```python
from build123d import *

# Parameters (mm, degrees)
F0_W     = 152.4
F0_H     = 177.8
F1_DEPTH = 88.9
F2_SIZE2 = 69.85
F2_SIZE  = 101.6
F3_W     = 127
F3_H     = 63.5
F4_DEPTH = 76.2


with BuildPart() as f1:
    # F0 (on Top) → F1 (new body)
    with BuildSketch(Plane.XY):
        with Locations((1.3535544276, 18.5724278663)):
            Rectangle(F0_W, F0_H)
    extrude(amount=F1_DEPTH)

    # F2
    f2_edges = [f1.edges().sort_by_distance(p)[0] for p in [
        (1.353554, -70.327572, 88.9),
    ]]
    f2_side = f1.faces().sort_by_distance((1.353554, 18.572428, 88.9))[0]
    chamfer(f2_edges, length=F2_SIZE, length2=F2_SIZE2, reference=f2_side)

    # F3 (on face) → F4 (cut)
    with BuildSketch(Plane(origin=(0, 107.4724278663, 0), x_dir=(-1, 0, 0), z_dir=(0, 1, 0))):
        with Locations((-1.3535544276, 44.45)):
            Rectangle(F3_W, F3_H)
    extrude(amount=-F4_DEPTH, mode=Mode.SUBTRACT)


solid = f1.part
```
Model file for the job. Use its own axes, mm. A direction names the side the tool comes from. Give positions to 0.01 mm unless a question says otherwise; leave off trailing zeros. Loops run counter-clockwise (first coordinate to the right, second up) from the corner with the lowest first, then second, coordinate; pieces in that order, holes last. Notation, with made-up numbers: (35.5, 49) -> (51.5, 49) arc R6 ccw to (51.5, 55) -> close; hole circle Ø9 at (73, -8). An arc over 180 degrees is marked (long way). Use CSV: the item, a comma, the result in double quotes. Start each with the question number.
1) Tool access for faces 1 (the flat face through (0, 20, 0)), 2 (the flat face through (2, 70, 76.2)): list every direction of +Z, -Z, +X, -X, +Y, -Y with a clear straight run to the whole face (end or side of a thin tool).
2) Slice it at C-C on z = 21.5. Give the cut face in (x, y).
3) Flat gauge pins, fed straight in: pin 1 Ø6 at (x, z) = (45.5, 78) entering from -Y; pin 2 Ø12 at (x, y) = (-6, -52.5) entering from +Z; pin 3 Ø10 at (x, y) = (20, -21) entering from -Z. Where does each tip first touch, or does it go through?
4) Slice it at A-A on y = 87.5. Give the cut face in (x, z), plus the area to 3 significant figures.
5) Wall check: line 1 (Z direction, x = -36, y = 99); line 2 (X direction, y = 76.5, z = 30.5); line 3 (Y direction, x = 31, z = 23). Give the ranges that are in metal, low to high.
6) Slice it at B-B on x = -29. Give the cut face in (y, z), plus the area to 3 significant figures.
7) Mould opens along X. For faces 3 (the flat face through (2, 31.272, 45)), 4 (the flat face through (0, 107.472, 4)), 5 (the flat face through (77.554, 37, 34)) say: released by +X, released by -X, zero draft, split by the parting line, or undercut.
8) Slice it at D-D on y = 27. Give the cut face in (x, z).
Computed values:
1,face 1,"-Z, +X, -X, +Y, -Y"
1,face 2,"+Y"
2,outline,"(-74.85, -66.76) -> (77.55, -66.76) -> (77.55, 107.47) -> (64.85, 107.47) -> (64.85, 31.27) -> (-62.15, 31.27) -> (-62.15, 107.47) -> (-74.85, 107.47) -> close"
3,pin 1,"stops at y = 11.05"
3,pin 2,"stops at z = 35.43"
3,pin 3,"stops at z = 0"
4,outline,"(-74.85, 0) -> (77.55, 0) -> (77.55, 88.9) -> (-74.85, 88.9) -> close; hole (-62.15, 12.7) -> (64.85, 12.7) -> (64.85, 76.2) -> (-62.15, 76.2) -> close"
4,area,"5,480 mm^2"
5,line 1,"z = 0 to 12.7, 76.2 to 88.9"
5,line 2,"x = -74.85 to -62.15, 64.85 to 77.55"
5,line 3,"y = -64.58 to 31.27"
6,outline,"(-70.33, 0) -> (107.47, 0) -> (107.47, 12.7) -> (31.27, 12.7) -> (31.27, 76.2) -> (107.47, 76.2) -> (107.47, 88.9) -> (31.27, 88.9) -> (-70.33, 19.05) -> close"
6,area,"7,420 mm^2"
7,face 3,"undercut"
7,face 4,"zero draft"
7,face 5,"released by +X"
8,outline,"(-74.85, 0) -> (77.55, 0) -> (77.55, 85.96) -> (-74.85, 85.96) -> close"
